from build123d import *

# Parameters (mm, degrees)
F0_W         = 76.2
F0_H         = 63.5
F1_DEPTH     = 15.24
F2_W         = 76.2
F2_H         = 8.89
F3_DEPTH     = 8.89
F4_R         = 5.08
F5_T1_DEPTH  = 16.51
F5_T3_DEPTH  = 49.53
F5_T5_DEPTH  = 66.04
F5_T7_DEPTH  = 22.86
F5_S11_W     = 5.08
F5_S11_H     = 5.08
F5_T12_DEPTH = 5.08
F5_S17_W     = 5.08
F5_S17_H     = 5.08
F5_T18_DEPTH = 5.08
F5_S23_W     = 5.08
F5_S23_H     = 5.08
F5_T24_DEPTH = 5.08
F5_S29_W     = 5.08
F5_S29_H     = 5.08
F5_T30_DEPTH = 5.08
F6_R         = 1.27


# Not quite as in the source:
# - a fillet or chamfer that OpenCascade refuses, or shapes differently, is made with other operations: its cross-section is extruded or revolved along the edge and cut away or added


with BuildPart() as f1:
    # F0 (on Top) → F1 (new body)
    with BuildSketch(Plane.XY):
        Rectangle(F0_W, F0_H)
    extrude(amount=F1_DEPTH)

    # F2 (on face) → F3 (join)
    with BuildSketch(Plane.XY.offset(15.24)):
        with Locations((0, -27.305)):
            Rectangle(F2_W, F2_H)
    extrude(amount=F3_DEPTH)

    # F4
    f4_edges = [f1.edges().sort_by_distance(p)[0] for p in [
        (38.1, -31.75, 12.065),
        (-38.1, -31.75, 12.065),
        (0, -31.75, 24.13),
    ]]
    fillet(f4_edges, radius=F4_R)

    # F5: fillet of radius 5.08 on 7 edges, made by hand

    # F5_s2 → F5_t1 (cut)
    with BuildSketch(Plane.XZ.offset(10.16)):
        with BuildLine():
            ThreePointArc((-33.02, 24.13), (-36.6121024484, 22.6421024484), (-38.1, 19.05))
            Line((-38.1, 19.05), (-38.1, 24.13))
            Line((-38.1, 24.13), (-33.02, 24.13))
        make_face()
        with BuildLine():
            ThreePointArc((38.1, 19.05), (36.6121024484, 22.6421024484), (33.02, 24.13))
            Line((33.02, 24.13), (38.1, 24.13))
            Line((38.1, 24.13), (38.1, 19.05))
        make_face()
    extrude(amount=F5_T1_DEPTH, mode=Mode.SUBTRACT)

    # F5_s4 → F5_t3 (cut)
    with BuildSketch(Plane.XZ.offset(-26.67)):
        with BuildLine():
            ThreePointArc((-33.02, 15.24), (-36.6121024484, 13.7521024484), (-38.1, 10.16))
            Line((-38.1, 10.16), (-38.1, 15.24))
            Line((-38.1, 15.24), (-33.02, 15.24))
        make_face()
        with BuildLine():
            ThreePointArc((38.1, 10.16), (36.6121024484, 13.7521024484), (33.02, 15.24))
            Line((33.02, 15.24), (38.1, 15.24))
            Line((38.1, 15.24), (38.1, 10.16))
        make_face()
    extrude(amount=F5_T3_DEPTH, mode=Mode.SUBTRACT)

    # F5_s6 → F5_t5 (cut)
    with BuildSketch(Plane.YZ.offset(-33.02)):
        with BuildLine():
            ThreePointArc((26.67, 15.24), (30.2621024484, 13.7521024484), (31.75, 10.16))
            Line((31.75, 10.16), (31.75, 15.24))
            Line((31.75, 15.24), (26.67, 15.24))
        make_face()
    extrude(amount=F5_T5_DEPTH, mode=Mode.SUBTRACT)

    # F5_s8 → F5_t7 (cut)
    with BuildSketch(Plane.XY.offset(-12.7)):
        with BuildLine():
            ThreePointArc((38.1, 26.67), (36.6121024484, 30.2621024484), (33.02, 31.75))
            Line((33.02, 31.75), (38.1, 31.75))
            Line((38.1, 31.75), (38.1, 26.67))
        make_face()
        with BuildLine():
            ThreePointArc((-33.02, 31.75), (-36.6121024484, 30.2621024484), (-38.1, 26.67))
            Line((-38.1, 26.67), (-38.1, 31.75))
            Line((-38.1, 31.75), (-33.02, 31.75))
        make_face()
    extrude(amount=F5_T7_DEPTH, mode=Mode.SUBTRACT)


with BuildPart() as f5_tool10:
    # F5_s11 → F5_t12 (new body)
    with BuildSketch(Plane.YZ.offset(33.02)):
        with Locations((-29.21, 21.59)):
            Rectangle(F5_S11_W, F5_S11_H)
    extrude(amount=F5_T12_DEPTH)

    # F5_s13 → F5_t14 (revolve, cut)
    with BuildSketch(Plane(origin=(33.02, -26.67, 19.05), x_dir=(0, 0.7071067812, -0.7071067812), z_dir=(0, -0.7071067812, -0.7071067812))):
        with BuildLine():
            ThreePointArc((0, -5.08), (5.08, 0), (0, 5.08))
            Line((0, 5.08), (0, -5.08))
        make_face()
    revolve(axis=Axis((33.02, -26.67, 19.05), (1, 0, 0)), mode=Mode.SUBTRACT)


with BuildPart() as f1_1:
    add(f1.part)

    # F5_t9: cut F5_tool10
    add(f5_tool10.part, mode=Mode.SUBTRACT)


with BuildPart() as f5_tool16:
    # F5_s17 → F5_t18 (new body)
    with BuildSketch(Plane.XY.offset(19.05)):
        with Locations((-35.56, -29.21)):
            Rectangle(F5_S17_W, F5_S17_H)
    extrude(amount=F5_T18_DEPTH)

    # F5_s19 → F5_t20 (revolve, cut)
    with BuildSketch(Plane(origin=(-33.02, -26.67, 19.05), x_dir=(0.7071067812, 0.7071067812, 0), z_dir=(0.7071067812, -0.7071067812, 0))):
        with BuildLine():
            ThreePointArc((0, -5.08), (5.08, 0), (0, 5.08))
            Line((0, 5.08), (0, -5.08))
        make_face()
    revolve(axis=Axis((-33.02, -26.67, 19.05), (0, 0, 1)), mode=Mode.SUBTRACT)


with BuildPart() as f1_2:
    add(f1_1.part)

    # F5_t15: cut F5_tool16
    add(f5_tool16.part, mode=Mode.SUBTRACT)


with BuildPart() as f5_tool22:
    # F5_s23 → F5_t24 (new body)
    with BuildSketch(Plane.XY.offset(10.16)):
        with Locations((-35.56, 29.21)):
            Rectangle(F5_S23_W, F5_S23_H)
    extrude(amount=F5_T24_DEPTH)

    # F5_s25 → F5_t26 (revolve, cut)
    with BuildSketch(Plane(origin=(-33.02, 26.67, 10.16), x_dir=(0.7071067812, -0.7071067812, 0), z_dir=(-0.7071067812, -0.7071067812, 0))):
        with BuildLine():
            ThreePointArc((0, -5.08), (5.08, 0), (0, 5.08))
            Line((0, 5.08), (0, -5.08))
        make_face()
    revolve(axis=Axis((-33.02, 26.67, 10.16), (0, 0, 1)), mode=Mode.SUBTRACT)


with BuildPart() as f1_3:
    add(f1_2.part)

    # F5_t21: cut F5_tool22
    add(f5_tool22.part, mode=Mode.SUBTRACT)


with BuildPart() as f5_tool28:
    # F5_s29 → F5_t30 (new body)
    with BuildSketch(Plane.YZ.offset(33.02)):
        with Locations((29.21, 12.7)):
            Rectangle(F5_S29_W, F5_S29_H)
    extrude(amount=F5_T30_DEPTH)

    # F5_s31 → F5_t32 (revolve, cut)
    with BuildSketch(Plane(origin=(33.02, 26.67, 10.16), x_dir=(0, -0.7071067812, -0.7071067812), z_dir=(0, -0.7071067812, 0.7071067812))):
        with BuildLine():
            ThreePointArc((0, -5.08), (5.08, 0), (0, 5.08))
            Line((0, 5.08), (0, -5.08))
        make_face()
    revolve(axis=Axis((33.02, 26.67, 10.16), (1, 0, 0)), mode=Mode.SUBTRACT)


with BuildPart() as f1_4:
    add(f1_3.part)

    # F5_t27: cut F5_tool28
    add(f5_tool28.part, mode=Mode.SUBTRACT)

    # F6
    f6_edges = [f1_4.edges().sort_by_distance(p)[0] for p in [
        (38.1, -22.86, 14.605),
        (36.612102, -22.86, 22.642102),
        (-38.1, -22.86, 14.605),
        (-36.612102, -22.86, 22.642102),
        (0, -22.86, 24.13),
    ]]
    fillet(f6_edges, radius=F6_R)


solid = f1_4.part
Check sheet for the modelled part. Datum: model origin and axes. Units: mm. A direction names the side the tool comes from. Round coordinates to 2 decimals unless told otherwise and drop trailing zeros. Write each loop counter-clockwise with the first axis right and the second up, starting at its lowest first coordinate (ties: lowest second). Pieces come first, ordered by that corner, then holes. Notation, with made-up numbers: (47, 22) - (76, 22) arc R20 cw to (76, 60) - close; hole circle Ø4 at (-36, -22.75). An arc over 180 degrees is marked (long way). Return JSON: item names as keys, results as strings.
Q1. Cross-section at C-C (z = 12). Record the boundary of the cut face in (x, y), then the cut area to 3 significant figures.
Returned:
{"outline": "(-38.1, -26.67) arc R5.08 ccw to (-33.02, -31.75) - (33.02, -31.75) arc R5.08 ccw to (38.1, -26.67) - (38.1, -24.13) arc R1.27 ccw to (37.76, -23.26) - (37.76, 26.67) arc R4.74 ccw to (33.02, 31.41) - (-33.02, 31.41) arc R4.74 ccw to (-37.76, 26.67) - (-37.76, -23.26) arc R1.27 ccw to (-38.1, -24.13) - close", "area": "4,750 mm²"}
Q2. Depth check by flat-ended pin: P1, Ø10.5, axis at x = -17, z = 19.5, coming from the +Y side; P2, Ø8, axis at x = -1, y = -17.5, coming from the +Z side. Enter the tip coordinate at first touch or a pass-through.
Returned:
{"P1": "stops at y = 29.68", "P2": "stops at z = 15.24"}
Q3. Access from +Z, -Z, +X, -X, +Y, -Y to the whole of each face (thin tool, end or side, straight path). Record for faces 1 (the cylindrical face through (36.651, 1.626, 13.712)), 2 (the flat face through (0, 2, 15.24)), 3 (the flat face through (38.1, 0, 5)), 4 (the cylindrical face through (-36.572, 1.626, 13.791)), 5 (the flat face through (-1, 0, 0)).
Returned:
{"face 1": "+Z, +X, +Y", "face 2": "+Z, +X, -X, +Y", "face 3": "+Z, -Z, +X, +Y, -Y", "face 4": "+Z, -X, +Y", "face 5": "-Z, +X, -X, +Y, -Y"}
Q4. Cross-section at A-A (x = 23). Record the boundary of the cut face in (y, z).
Returned:
{"outline": "(-31.75, 0) - (31.75, 0) - (31.75, 10.16) arc R5.08 ccw to (26.67, 15.24) - (-22.86, 15.24) - (-22.86, 22.86) arc R1.27 ccw to (-24.13, 24.13) - (-26.67, 24.13) arc R5.08 ccw to (-31.75, 19.05) - close"}
Q5. Cross-section at B-B (y = -10). Record the boundary of the cut face in (x, z), then the cut area to 3 significant figures.
Returned:
{"outline": "(-38.1, 0) - (38.1, 0) - (38.1, 10.16) arc R5.08 ccw to (33.02, 15.24) - (-33.02, 15.24) arc R5.08 ccw to (-38.1, 10.16) - close", "area": "1,150 mm²"}
Q6. Scan lines: L1, parallel to Z at x = -19, y = -14; L2, parallel to Y at x = 27, z = 18.5; L3, parallel to Y at x = -20.5, z = 20. Record each from-to range of solid material in increasing order. Write a range as from..to.
Returned:
{"L1": "z = 0..15.24", "L2": "y = -31.75..-22.86", "L3": "y = -31.66..-22.86"}
